Geometry check sheet. Reference: drawing and pictorial views, mm from the part's lowest x, y, z. A direction names the side the tool comes from. Coordinates: 2 decimals unless noted, no trailing zeros. Write each loop counter-clockwise with the first axis right and the second up, starting at its lowest first coordinate (ties: lowest second). Pieces come first, ordered by that corner, then holes. Notation, with made-up numbers: (18.5, 71) - (45.5, 71) arc R6 cw to (45.5, 76) - close; hole circle Ø2 at (-25, -16). An arc over 180 degrees is marked (long way). Use one line per item in the form item = value. Start each with the question number.
(1) Tool access check on the marked faces 1, 2, 3 and 4. Record the directions out of +Z, -Z, +X, -X, +Y, -Y that give a thin tool (end or side, any length) a straight path to the whole face; none if there is none.
(2) Material ranges on line 1 (X direction, y = 24.5, z = 1.5); line 2 (Y direction, x = 6, z = 13.5), recorded low to high. Write a range as [from, to].
(3) Gauge pin test, flat ends, axial feed: pin 1 Ø3 at (y, z) = (34, 7.5) entering from +X; pin 2 Ø6.5 at (x, z) = (53, 7) entering from +Y; pin 3 Ø6 at (x, y) = (6.5, 16.5) entering from +Z; pin 4 Ø8 at (y, z) = (32.5, 6.5) entering from -X. Record the tip position at first contact, or that the pin passes through.
(4) Sectioned sample at C-C (x = 50). Record the cut outline in (y, z), and give its area (3 significant figures).
(5) Sectioned sample at B-B (y = 33). Record the cut outline in (x, z), and give its area (3 significant figures).
(6) Sectioned sample at A-A (z = 3.75). Record the cut outline in (x, y).
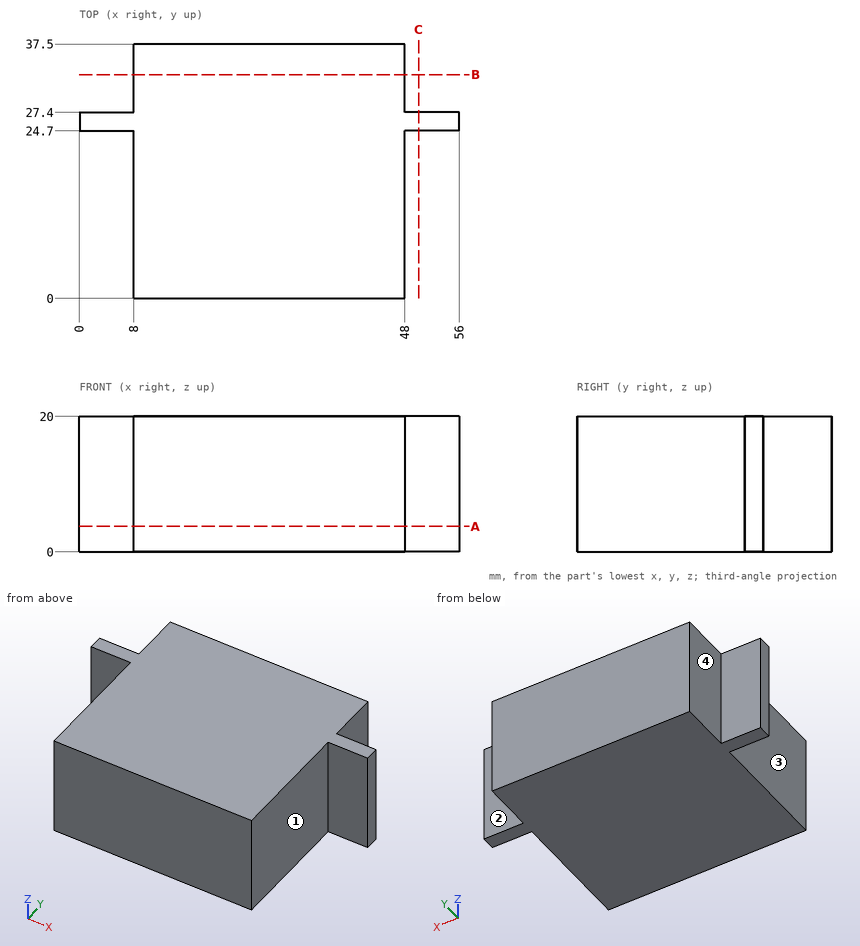
Answers below:
q1.face_1 = +Z, -Z, +X, -Y
q1.face_2 = +Z, -Z, +X, +Y
q1.face_3 = +Z, -Z, -X, -Y
q1.face_4 = +Z, -Z, -X, +Y
q2.line_1 = [8, 48]
q2.line_2 = [24.7, 27.4]
q3.pin_1 = 48
q3.pin_2 = 27.4
q3.pin_3 = 20
q3.pin_4 = 8
q4.outline = (24.7, 0) - (27.4, 0) - (27.4, 20) - (24.7, 20) - close
q4.area = 54.0 mm2
q5.outline = (8, 0) - (48, 0) - (48, 20) - (8, 20) - close
q5.area = 800 mm2
q6.outline = (0, 24.7) - (8, 24.7) - (8, 0) - (48, 0) - (48, 24.7) - (56, 24.7) - (56, 27.4) - (48, 27.4) - (48, 37.5) - (8, 37.5) - (8, 27.4) - (0, 27.4) - close
